from build123d import *

# Parameters (mm, degrees)
SKETCH1_R           = 1.499976783
BOSS_EXTRUDE1_DEPTH = 3.175


with BuildPart() as part:
    # Sketch1 → Boss-Extrude1 (new body)
    with BuildSketch(Plane(origin=(0, 0, 0), x_dir=(1, 0, 0), z_dir=(0, 1, 0))):
        with BuildLine():
            Line((29.861952869, -5.757321993), (26.667645588, -5.757321993))
            Line((26.667645588, -5.757321993), (26.667645588, -0.857080759))
            add(Edge.make_bspline(
                [(26.667645588, -0.857080759), (25.72356302, 9.922922576), (25.103649505, 12.257419962), (25.095153567, 12.168136444)],
                knots=[3, 3, 3, 3, 4, 4, 4, 4], degree=3))
            add(Edge.make_bspline(
                [(25.095153567, 12.168136444), (24.467255917, 14.632886979), (21.327316795, 17.843284785), (17.583634713, 17.647304435)],
                knots=[4, 4, 4, 4, 5, 5, 5, 5], degree=3))
            add(Edge.make_bspline(
                [(17.583634713, 17.647304435), (14.112817036, 17.647304435), (11.16518444, 15.401572953), (10.109869901, 12.281874779)],
                knots=[5, 5, 5, 5, 6, 6, 6, 6], degree=3))
            add(Edge.make_bspline(
                [(10.109869901, 12.281874779), (8.875160908, 9.099252332), (8.353569729, -0.584552145), (-21.846222224, -0.989511791)],
                knots=[6, 6, 6, 6, 7, 7, 7, 7], degree=3))
            Line((-21.846222224, -0.989511791), (-21.74662038, -0.989511791))
            Line((-21.74662038, -0.989511791), (-21.74662038, -8.05752013))
            Line((-21.74662038, -8.05752013), (-24.242242708, -8.05752013))
            Line((-24.242242708, -8.05752013), (-24.242242708, -14.557549737))
            Line((-24.242242708, -14.557549737), (-21.225926076, -14.557549737))
            Line((-21.225926076, -14.557549737), (-21.225926076, -16.957715728))
            Line((-21.225926076, -16.957715728), (-18.530788103, -16.957715728))
            Line((-18.530788103, -16.957715728), (-18.530788103, -14.557549737))
            Line((-18.530788103, -14.557549737), (-17.354341851, -14.557549737))
            Line((-17.354341851, -14.557549737), (-17.354341851, -16.957715728))
            Line((-17.354341851, -16.957715728), (-11.742742556, -16.957715728))
            Line((-11.742742556, -16.957715728), (-11.742742556, -14.557549737))
            Line((-11.742742556, -14.557549737), (-4.290380881, -14.557549737))
            Line((-4.290380881, -14.557549737), (-4.277541923, -14.557549737))
            Line((-4.277541923, -14.557549737), (-4.277541923, -10.857323134))
            Line((-4.277541923, -10.857323134), (10.695923955, -10.857323134))
            Line((10.695923955, -10.857323134), (10.695923955, -14.557422775))
            Line((10.695923955, -14.557422775), (16.724267817, -14.557422775))
            Line((16.724267817, -14.557422775), (16.724267817, -16.957715728))
            Line((16.724267817, -16.957715728), (25.708547678, -16.957715728))
            Line((25.708547678, -16.957715728), (25.708547678, -14.557549737))
            Line((25.708547678, -14.557549737), (29.861952869, -14.557549737))
            Line((29.861952869, -14.557549737), (29.861952869, -5.757321993))
        make_face()
        with Locations(Location((17.58369808, 9.243227132, 0), (0, 0, 270))):
            Circle(SKETCH1_R, mode=Mode.SUBTRACT)
    extrude(amount=BOSS_EXTRUDE1_DEPTH)


solid = part.part
Verification items for the finished model (mm, model axes). A direction names the side the tool comes from. Coordinates: 2 decimals unless noted, no trailing zeros. Order: outer loops, then holes, each group sorted by start corner. A loop starts at its lowest first (then second) coordinate and runs counter-clockwise, first axis right, second up. Notation, with made-up numbers: M 31.25,26.25 L 38.25,26.25 A21 ccw 38.25,61.25 Z; hole C -32.75,43.25 d2. An arc over 180 degrees is marked long. One line per item, written item: value. Start each with the question number.
Item 1: Mould release check, pull along X, two halves, no side actions. Record for faces 1 (the flat face through (16.724, 2, 16)), 2 (the flat face through (8, 0, 3)), 3 (the flat face through (25.709, 2, 16)): pulls with the +X half, pulls with the -X half, needs draft (parallel to the pull), parting line crosses it, or undercut.
Item 2: Access from +Z, -Z, +X, -X, +Y, -Y to the whole of each face (thin tool, end or side, straight path). Record for faces 4 (the flat face through (-17.354, 2, 16)), 5 (the flat face through (-21.747, 2, 4)), 6 (the flat face through (26.668, 2, 3)), 7 (the flat face through (-21.226, 2, 16)).
Item 3: Depth check by flat-ended pin: P1, Ø1, axis at x = 19.5, y = 1.5, coming from the -Z side; P2, Ø1, axis at y = 1.5, z = 2, coming from the +X side; P3, Ø1.2, axis at y = 2, z = 16, coming from the -X side. Enter the tip coordinate at first touch or a pass-through.
Item 4: Sectioned sample at A-A on z = 4. Record the cut outline in (x, y) (3 decimals).
Item 5: Thickness scan on probe 1 along X at (y, z) = (0.65, 11); probe 2 along X at (y, z) = (1.2, 6.5); probe 3 along X at (y, z) = (1.8, -10.5). Record the ranges inside material, lowest first.
Calculated:
1. face 1: undercut
1. face 2: needs draft
1. face 3: pulls with the +X half
2. face 4: +Z, +Y, -Y
2. face 5: -X, +Y, -Y
2. face 6: -Z, +X, +Y, -Y
2. face 7: +Z, -X, +Y, -Y
3. P1: z = -17.56
3. P2: x = 26.67
3. P3: x = -21.23
4. outline: M -21.747,0 L 26.668,0 L 26.668,3.175 L -21.747,3.175 Z
5. probe 1: -24.24 to -4.28, 10.7 to 29.86
5. probe 2: -21.75 to 29.86
5. probe 3: 9.51 to 16.76, 18.4 to 25.42
